Verification items for the finished model (mm, model axes). A direction names the side the tool comes from. Give positions to 0.01 mm unless a question says otherwise; leave off trailing zeros. Order: outer loops, then holes, each group sorted by start corner. A loop starts at its lowest first (then second) coordinate and runs counter-clockwise, first axis right, second up. Notation, with made-up numbers: M -5,-9 L 38,-9 A29 ccw 38,14 Z; hole C 36.25,87 d9. An arc over 180 degrees is marked long. Answer as a JSON object with one key per item and string values.
```python
from build123d import *

# Parameters (mm, degrees)
SKETCH2_W           = 50.8
SKETCH2_H           = 25.4
SKETCH2_W_2         = 45.72
SKETCH2_H_2         = 20.32
BOSS_EXTRUDE1_DEPTH = 635
SKETCH3_R           = 2.032
CUT_EXTRUDE1_DEPTH  = 638.155342126
SKETCH6_W           = 50.8
SKETCH6_H           = 25.4
CUT_EXTRUDE4_DEPTH  = 571.5


with BuildPart() as part:
    # Sketch2 → Boss-Extrude1 (new body)
    with BuildSketch(Plane(origin=(0, 0, 0), x_dir=(1, 0, 0), z_dir=(0, 1, 0))):
        Rectangle(SKETCH2_W, SKETCH2_H)
        Rectangle(SKETCH2_W_2, SKETCH2_H_2, mode=Mode.SUBTRACT)
    extrude(amount=BOSS_EXTRUDE1_DEPTH)

    # Sketch3 → Cut-Extrude1 (cut, through all)
    with BuildSketch(Plane(origin=(25.4, 0, 0), x_dir=(0, 0, -1), z_dir=(1, 0, 0))):
        Circle(SKETCH3_R)
        with Locations((0, 12.7)):
            Circle(SKETCH3_R)
        with Locations((0, 25.4)):
            Circle(SKETCH3_R)
        with Locations((0, 38.1)):
            Circle(SKETCH3_R)
        with Locations((0, 50.8)):
            Circle(SKETCH3_R)
        with Locations((0, 63.5)):
            Circle(SKETCH3_R)
        with Locations((0, 76.2)):
            Circle(SKETCH3_R)
        with Locations((0, 88.9)):
            Circle(SKETCH3_R)
        with Locations((0, 101.6)):
            Circle(SKETCH3_R)
        with Locations((0, 114.3)):
            Circle(SKETCH3_R)
        with Locations((0, 127)):
            Circle(SKETCH3_R)
        with Locations((0, 139.7)):
            Circle(SKETCH3_R)
        with Locations((0, 152.4)):
            Circle(SKETCH3_R)
        with Locations((0, 165.1)):
            Circle(SKETCH3_R)
        with Locations((0, 177.8)):
            Circle(SKETCH3_R)
        with Locations((0, 190.5)):
            Circle(SKETCH3_R)
        with Locations((0, 203.2)):
            Circle(SKETCH3_R)
        with Locations((0, 215.9)):
            Circle(SKETCH3_R)
        with Locations((0, 228.6)):
            Circle(SKETCH3_R)
        with Locations((0, 241.3)):
            Circle(SKETCH3_R)
        with Locations((0, 254)):
            Circle(SKETCH3_R)
        with Locations((0, 266.7)):
            Circle(SKETCH3_R)
        with Locations((0, 279.4)):
            Circle(SKETCH3_R)
        with Locations((0, 292.1)):
            Circle(SKETCH3_R)
        with Locations((0, 304.8)):
            Circle(SKETCH3_R)
        with Locations((0, 317.5)):
            Circle(SKETCH3_R)
        with Locations((0, 330.2)):
            Circle(SKETCH3_R)
        with Locations((0, 342.9)):
            Circle(SKETCH3_R)
        with Locations((0, 355.6)):
            Circle(SKETCH3_R)
        with Locations((0, 368.3)):
            Circle(SKETCH3_R)
        with Locations((0, 381)):
            Circle(SKETCH3_R)
        with Locations((0, 393.7)):
            Circle(SKETCH3_R)
        with Locations((0, 406.4)):
            Circle(SKETCH3_R)
        with Locations((0, 419.1)):
            Circle(SKETCH3_R)
        with Locations((0, 431.8)):
            Circle(SKETCH3_R)
        with Locations((0, 444.5)):
            Circle(SKETCH3_R)
        with Locations((0, 457.2)):
            Circle(SKETCH3_R)
        with Locations((0, 469.9)):
            Circle(SKETCH3_R)
        with Locations((0, 482.6)):
            Circle(SKETCH3_R)
        with Locations((0, 495.3)):
            Circle(SKETCH3_R)
        with Locations((0, 508)):
            Circle(SKETCH3_R)
        with Locations((0, 520.7)):
            Circle(SKETCH3_R)
        with Locations((0, 533.4)):
            Circle(SKETCH3_R)
        with Locations((0, 546.1)):
            Circle(SKETCH3_R)
        with Locations((0, 558.8)):
            Circle(SKETCH3_R)
        with Locations((0, 571.5)):
            Circle(SKETCH3_R)
        with Locations((0, 584.2)):
            Circle(SKETCH3_R)
        with Locations((0, 596.9)):
            Circle(SKETCH3_R)
        with Locations((0, 609.6)):
            Circle(SKETCH3_R)
        with Locations((0, 622.3)):
            Circle(SKETCH3_R)
    extrude(amount=-CUT_EXTRUDE1_DEPTH, mode=Mode.SUBTRACT)

    # Sketch6 → Cut-Extrude4 (cut)
    with BuildSketch(Plane(origin=(0, 635, 0), x_dir=(1, 0, 0), z_dir=(0, 1, 0))):
        Rectangle(SKETCH6_W, SKETCH6_H)
    extrude(amount=-CUT_EXTRUDE4_DEPTH, mode=Mode.SUBTRACT)


solid = part.part
```
Q1. Gauge pin test, flat end, axial feed: pin 1 Ø3.5 at (y, z) = (12.7, 0) entering from +X. Record the tip position at first contact, or that the pin passes through.
Resolved:
{"pin 1": "passes through"}
Q2. Section check B-B on y = 12.7. Record the cut outline in (x, z), then the cut area to 3 significant figures.
Resolved:
{"outline": "M -25.4,-12.7 L 25.4,-12.7 L 25.4,-2.03 L 22.86,-2.03 L 22.86,-10.16 L -22.86,-10.16 L -22.86,-2.03 L -25.4,-2.03 Z; M -25.4,2.03 L -22.86,2.03 L -22.86,10.16 L 22.86,10.16 L 22.86,2.03 L 25.4,2.03 L 25.4,12.7 L -25.4,12.7 Z", "area": "341 mm²"}
Q3. Material ranges on L1, parallel to Y at x = 24.55, z = 0; L2, parallel to X at y = 47.5, z = -7; L3, parallel to Z at x = 0, y = 21, recorded low to high.
Resolved:
{"L1": "y = 2.03 to 10.67, 14.73 to 23.37, 27.43 to 36.07, 40.13 to 48.77, 52.83 to 61.47", "L2": "x = -25.4 to -22.86, 22.86 to 25.4", "L3": "z = -12.7 to -10.16, 10.16 to 12.7"}
Q4. Section check C-C on z = -8.5. Record the cut outline in (x, y).
Resolved:
{"outline": "M -25.4,0 L -22.86,0 L -22.86,63.5 L -25.4,63.5 Z; M 22.86,0 L 25.4,0 L 25.4,63.5 L 22.86,63.5 Z"}
Q5. Section check D-D on y = 37. Record the cut outline in (x, z), then the cut area to 3 significant figures.
Resolved:
{"outline": "M -25.4,-12.7 L 25.4,-12.7 L 25.4,-1.71 L 22.86,-1.71 L 22.86,-10.16 L -22.86,-10.16 L -22.86,-1.71 L -25.4,-1.71 Z; M -25.4,1.71 L -22.86,1.71 L -22.86,10.16 L 22.86,10.16 L 22.86,1.71 L 25.4,1.71 L 25.4,12.7 L -25.4,12.7 Z", "area": "344 mm²"}
Q6. Release check for a two-part mould opening along Y. For faces 3 (the face through (-24.11, 2.03, -0.04)), 4 (the face through (-24.112, 48.816, 0.44)), 5 (the face through (24.15, 61.47, 0.04)) record: +Y half, -Y half, draft (parallel to the pull), parting line (faces both ways), or undercut.
Resolved:
{"face 3": "-Y half", "face 4": "undercut", "face 5": "+Y half"}
Q7. Tool access check on faces 1 (the face through (0, 31, -12.7)), 2 (the face through (0, 31, -10.16)). Record the directions out of +Z, -Z, +X, -X, +Y, -Y that give a thin tool (end or side, any length) a straight path to the whole face; none if there is none.
Resolved:
{"face 1": "-Z, +X, -X, +Y, -Y", "face 2": "+Y, -Y"}
Q8. Section check A-A on x = 17. Record the cut outline in (y, z).
Resolved:
{"outline": "M 0,-12.7 L 63.5,-12.7 L 63.5,-10.16 L 0,-10.16 Z; M 0,10.16 L 63.5,10.16 L 63.5,12.7 L 0,12.7 Z"}
